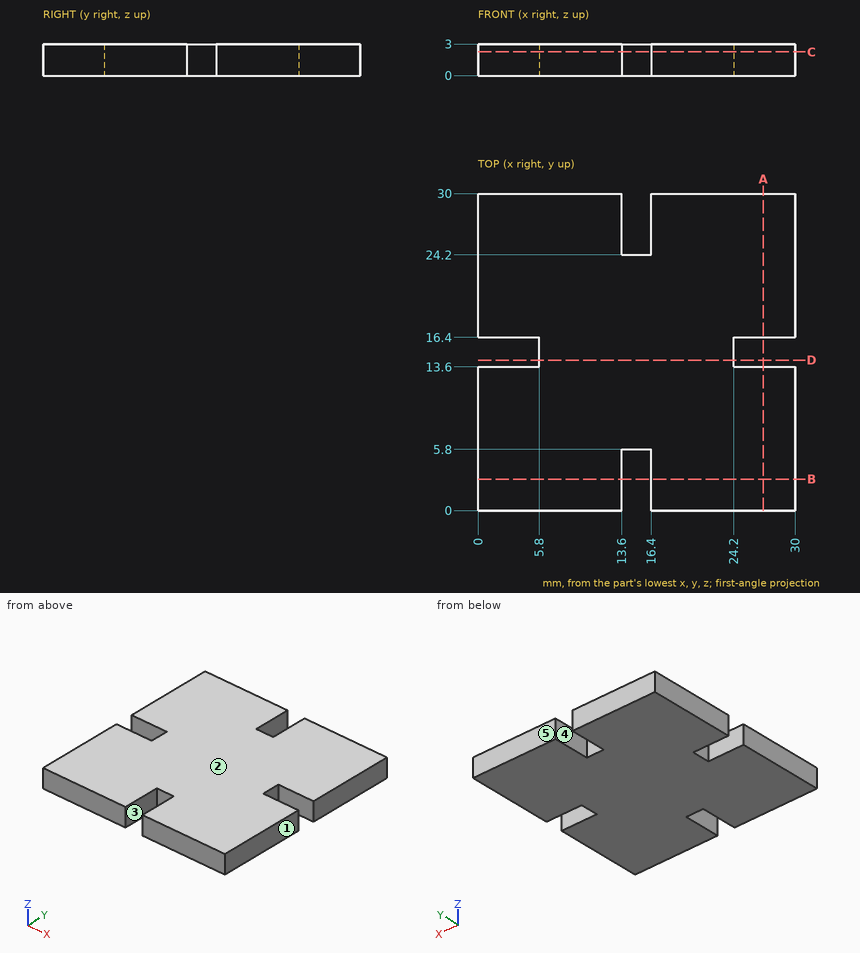
Geometry check sheet. Reference: drawing and pictorial views, mm from the part's lowest x, y, z. A direction names the side the tool comes from. Coordinates: 2 decimals unless noted, no trailing zeros. Loops run counter-clockwise (first coordinate to the right, second up) from the corner with the lowest first, then second, coordinate; pieces in that order, holes last. Notation, with made-up numbers: (57, 72) -> (88, 72) arc R24 cw to (88, 103) -> close; hole circle Ø1 at (14, 56.5). An arc over 180 degrees is marked (long way). Write item = value, one per line. Start each with the question number.
1. Tool access check on the marked faces 4 and 5. Record the directions out of +Z, -Z, +X, -X, +Y, -Y that give a thin tool (end or side, any length) a straight path to the whole face; none if there is none.
2. Section check A-A on x = 27. Record the cut outline in (y, z).
3. Material ranges on line 1 (Y direction, x = 3.5, z = 2.7); line 2 (X direction, y = 16, z = 2.7), recorded low to high.
4. Depth check by flat-ended pin: P1, Ø0.8, axis at x = 15.5, z = 1, coming from the +Y side; P2, Ø0.8, axis at x = 14.5, z = 2, coming from the -Y side; P3, Ø1.4, axis at y = 14.5, z = 1, coming from the -X side. Enter the tip coordinate at first touch or a pass-through.
5. Section check C-C on z = 2.25. Record the cut outline in (x, y), then the cut area to 3 significant figures.
6. Section check D-D on y = 14.25. Record the cut outline in (x, z).
7. Draft check along X on the marked faces 1, 2 and 3. Enter one of: released by +X, released by -X, zero draft, split by the parting line, or undercut.
Responses:
q1.face_4 = +Z, -Z, +Y
q1.face_5 = +Z, -Z, +X, -X, +Y
q2.outline = (0, 0) -> (13.6, 0) -> (13.6, 3) -> (0, 3) -> close; (16.4, 0) -> (30, 0) -> (30, 3) -> (16.4, 3) -> close
q3.line_1 = 0 to 13.6, 16.4 to 30
q3.line_2 = 5.8 to 24.2
q4.P1 = 24.2
q4.P2 = 5.8
q4.P3 = 5.8
q5.outline = (0, 0) -> (13.6, 0) -> (13.6, 5.8) -> (16.4, 5.8) -> (16.4, 0) -> (30, 0) -> (30, 13.6) -> (24.2, 13.6) -> (24.2, 16.4) -> (30, 16.4) -> (30, 30) -> (16.4, 30) -> (16.4, 24.2) -> (13.6, 24.2) -> (13.6, 30) -> (0, 30) -> (0, 16.4) -> (5.8, 16.4) -> (5.8, 13.6) -> (0, 13.6) -> close
q5.area = 835 mm2
q6.outline = (5.8, 0) -> (24.2, 0) -> (24.2, 3) -> (5.8, 3) -> close
q7.face_1 = released by +X
q7.face_2 = zero draft
q7.face_3 = undercut
